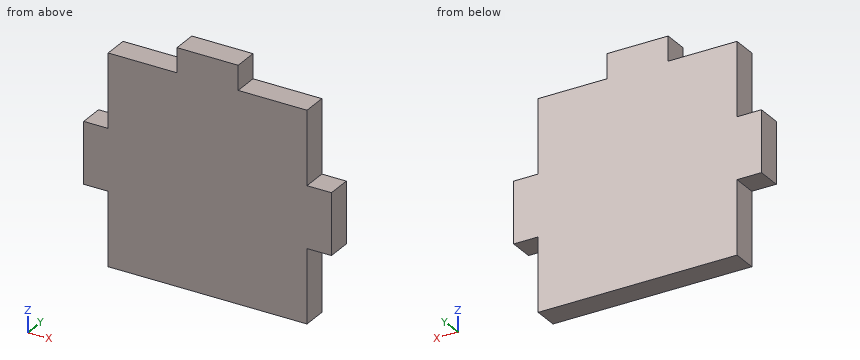
```python
from build123d import *

# Parameters (mm, degrees)
SKETCH1_W           = 32.5
SKETCH1_H           = 34
BOSS_EXTRUDE1_DEPTH = 4
SKETCH2_W           = 10
SKETCH2_H           = 4
SKETCH2_W_2         = 4
SKETCH2_H_2         = 10
BOSS_EXTRUDE2_DEPTH = 4


with BuildPart() as part:
    # Sketch1 → Boss-Extrude1 (new body)
    with BuildSketch(Plane(origin=(0, 0, 0), x_dir=(1, 0, 0), z_dir=(0, 1, 0))):
        with Locations((16.25, -17)):
            Rectangle(SKETCH1_W, SKETCH1_H)
    extrude(amount=BOSS_EXTRUDE1_DEPTH)

    # Sketch2 → Boss-Extrude2 (add, through all)
    with BuildSketch(Plane.XZ):
        with Locations((16.25, 36)):
            Rectangle(SKETCH2_W, SKETCH2_H)
        with Locations((34.5, 17)):
            Rectangle(SKETCH2_W_2, SKETCH2_H_2)
        with Locations((-2, 17)):
            Rectangle(SKETCH2_W_2, SKETCH2_H_2)
    extrude(amount=-BOSS_EXTRUDE2_DEPTH)


solid = part.part
```
The model under review builds one solid part; all positions refer to its coordinate system, in mm. Give positions to 0.01 mm unless a question says otherwise; leave off trailing zeros. Write each loop counter-clockwise with the first axis right and the second up, starting at its lowest first coordinate (ties: lowest second). Pieces come first, ordered by that corner, then holes. Notation, with made-up numbers: (-29.5, 7) - (-15.5, 7) arc R26 cw to (-15.5, 36) - close; hole circle Ø7 at (11, 18.5). An arc over 180 degrees is marked (long way). Answer in a Markdown table with one row per item. Add a question column.
1. We need section A-A on y = 2.3. Write out the cut boundary in (x, z).
2. We need section C-C on x = 27.5. Write out the cut boundary in (y, z), then the cut area to 3 significant figures.
3. We need section B-B on z = 3.5. Write out the cut boundary in (x, y).
4. Wall thickness on line 1 along Z through (x, y) = (27.5, 3.75); line 2 along X through (y, z) = (0.35, 27.5): over which ranges is each line inside the solid? List them lowest first. Write a range as [from, to].
5. Insertion check: P1, Ø2, axis at y = 1.5, z = 35.5, coming from the -X side; P2, Ø1.2, axis at x = 5.5, y = 1, coming from the +Z side; P3, Ø2, axis at y = 2, z = 26.5, coming from the -X side. Each pin has a flat end and moves straight along its axis. Give the tip position at first contact, or say it passes through.
Ans:
| question | item | result |
|---|---|---|
| 1 | outline | (-4, 12) - (0, 12) - (0, 0) - (32.5, 0) - (32.5, 12) - (36.5, 12) - (36.5, 22) - (32.5, 22) - (32.5, 34) - (21.25, 34) - (21.25, 38) - (11.25, 38) - (11.25, 34) - (0, 34) - (0, 22) - (-4, 22) - close |
| 2 | outline | (0, 0) - (4, 0) - (4, 34) - (0, 34) - close |
| 2 | area | 136 mm^2 |
| 3 | outline | (0, 0) - (32.5, 0) - (32.5, 4) - (0, 4) - close |
| 4 | line 1 | z = [0, 34] |
| 4 | line 2 | x = [0, 32.5] |
| 5 | P1 | stops at x = 11.25 |
| 5 | P2 | stops at z = 34 |
| 5 | P3 | stops at x = 0 |
